Geometry: see drawing. Coordinates: mm, zero at the bounding-box minimum. A direction names the side the tool comes from. Round coordinates to 2 decimals unless told otherwise and drop trailing zeros. Loops run counter-clockwise (first coordinate to the right, second up) from the corner with the lowest first, then second, coordinate; pieces in that order, holes last. Notation, with made-up numbers: M 18,45 L 61,45 A18 ccw 61,76 Z; hole C 56.25,14 d2. An arc over 180 degrees is marked long. Answer as a JSON object with one key per item and string values.
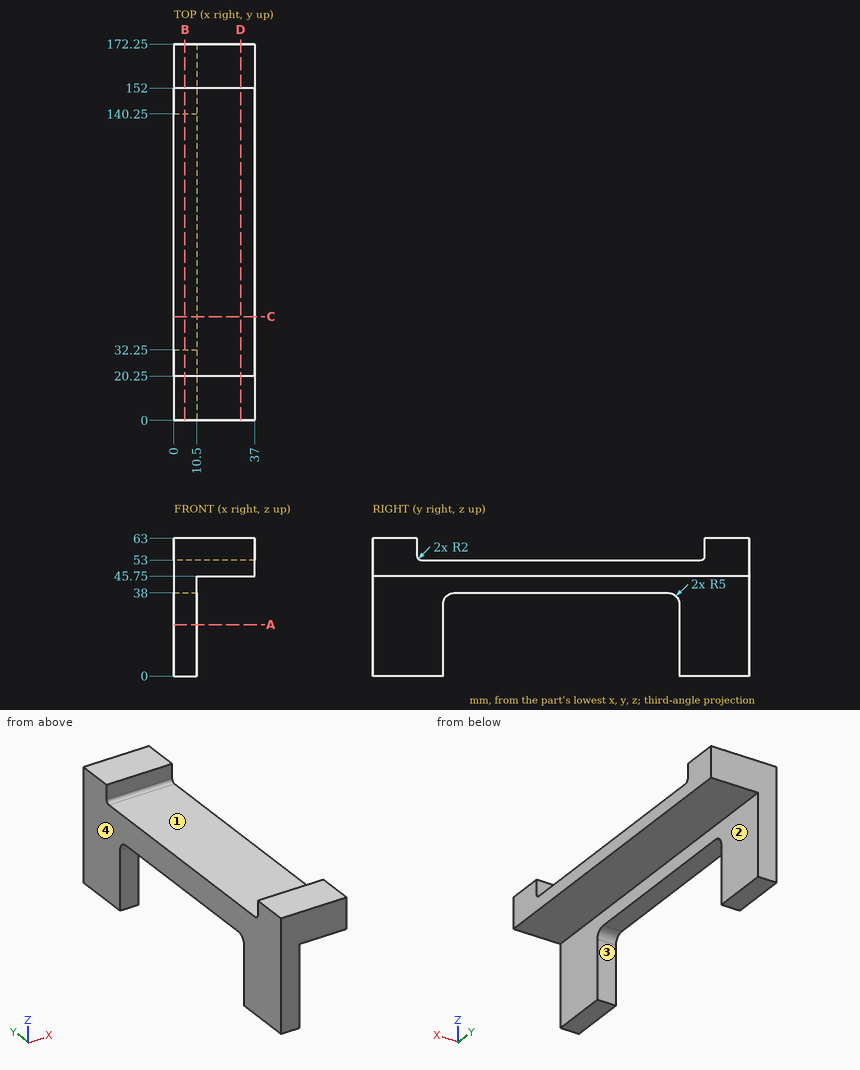
1) Reachability of the marked faces 1, 2, 3 and 4 from +Z, -Z, +X, -X, +Y, -Y: full face, straight path, thin tool, end or side. Return the list, or none.
Results:
{"face 1": "+Z, +X, -X", "face 2": "-Z, +X, +Y, -Y", "face 3": "-Z, +X, -X", "face 4": "+Z, -Z, -X, +Y, -Y"}
2) Pin query (flat end, axial travel): P1, Ø5, axis at x = 12, z = 34, coming from the -Y side; P2, Ø12, axis at x = 14, y = 127.5, coming from the -Z side; P3, Ø18.5, axis at x = 22, y = 117.5, coming from the +Z side; P4, Ø1, axis at y = 20, z = 33, coming from the +X side. Return the tip coordinate at first contact, or that it passes through.
Results:
{"P1": "y = 0", "P2": "z = 38", "P3": "z = 53", "P4": "x = 10.5"}
3) Section query C-C (y = 47.5). Return the cut outline in (x, z), and give its area (3 significant figures).
Results:
{"outline": "M 0,38 L 10.5,38 L 10.5,45.75 L 37,45.75 L 37,53 L 0,53 Z", "area": "350 mm2"}
4) Ray query, line 1 (Y direction, x = 4, z = 10.5); line 2 (Y direction, x = 12, z = 60.5); line 3 (Z direction, x = 14, y = 112). Return the intervals inside material, ascending.
Results:
{"line 1": "0 to 32.25, 140.25 to 172.25", "line 2": "0 to 20.25, 152 to 172.25", "line 3": "45.75 to 53"}
5) Section query A-A (z = 23.5). Return the cut outline in (x, y).
Results:
{"outline": "M 0,0 L 10.5,0 L 10.5,32.25 L 0,32.25 Z; M 0,140.25 L 10.5,140.25 L 10.5,172.25 L 0,172.25 Z"}
6) Section query D-D (x = 30.5). Return the cut outline in (y, z).
Results:
{"outline": "M 0,45.75 L 172.25,45.75 L 172.25,63 L 152,63 L 152,55 A2 cw 150,53 L 22.25,53 A2 cw 20.25,55 L 20.25,63 L 0,63 Z"}
7) Section query B-B (x = 5). Return the cut outline in (y, z).
Results:
{"outline": "M 0,0 L 32.25,0 L 32.25,33 A5 cw 37.25,38 L 135.25,38 A5 cw 140.25,33 L 140.25,0 L 172.25,0 L 172.25,63 L 152,63 L 152,55 A2 cw 150,53 L 22.25,53 A2 cw 20.25,55 L 20.25,63 L 0,63 Z"}
